Autodesk Inventor part; units mm, degrees
ref_plane "YZ Plane" through (0, 0, 0) normal (1, 0, 0) x (0, 1, 0)
ref_plane "XZ Plane" through (0, 0, 0) normal (0, 1, 0) x (-1, 0, 0)
ref_plane "XY Plane" through (0, 0, 0) normal (0, 0, 1) x (1, 0, 0)
sketch "Boceto1" plane through (0, 0, 0) normal (0, 1, 0) x (-1, 0, 0)
  arc A0 (16, 0) -> (-16, 0) centre (0, 0) ccw
  line L0 (0, 0) -> (45, 0) construction
  arc A1 (-16, -45) -> (16, -45) centre (0, -45) ccw
  line L1 (16, 0) -> (16, -45)
  line L2 (-16, -45) -> (-16, 0)
  arc A2 (15, 0) -> (-15, 0) centre (0, 0) ccw
  arc A3 (-15, -45) -> (15, -45) centre (0, -45) ccw
  line L3 (15, 0) -> (15, -45)
  line L4 (-15, -45) -> (-15, 0)
  dimension "d0" = 32
  dimension "d3" = 32
  dimension "d4" = 30
  dimension "d5" = 30
extrude "Extrusión1" add sketch "Boceto1" along normal blind 38
properties part number "Cinta"
CAD build for the part. Positions are in the model's coordinates, mm. A direction names the side the tool comes from. Give positions to 0.01 mm unless a question says otherwise; leave off trailing zeros. Loops run counter-clockwise (first coordinate to the right, second up) from the corner with the lowest first, then second, coordinate; pieces in that order, holes last. Notation, with made-up numbers: M 86,38.5 L 98,38.5 A6 ccw 98,42.5 Z; hole C 49,40.25 d11. An arc over 180 degrees is marked long. One line per question, with ' | ' between items. Start each with the question number.
1. Saw through at B-B on y = 3.5. Give the cut face in (x, z).
2. Two-plate mould, pull along Z, no slides. Class faces 3 (the face through (0, 19, 16)), 4 (the face through (0, 19, 15)), 5 (the face through (-15.3, 38, -19.5)): pulls with the +Z half, pulls with the -Z half, needs draft (parallel to the pull), parting line crosses it, or undercut.
3. Saw through at C-C on x = 7. Give the cut face in (y, z), plus the area to 3 significant figures.
4. Saw through at A-A on z = -38.5. Give the cut face in (x, y).
5. Probe L1, parallel to X at y = 17, z = -25; L2, parallel to Z at x = -5, y = 12; L3, parallel to X at y = 8.5, z = 2. List the from-to ranges inside material, lowest first. Write a range as from..to.
6. Flat gauge pins, fed straight in: pin 1 (12 mm diameter, centred on x = 13, y = 26, fed in from +Z); pin 2 (6 mm diameter, centred on x = -9.5, y = 4.5, fed in from +Z). Where does each tip first touch, or does it go through?
7. 3-axis set-ups, long thin cutter, end or side, ignore diameter. For faces 1 (the face through (16, 19, -23)), 2 (the face through (-15, 19, -22)): which of +Z, -Z, +X, -X, +Y, -Y reach the whole face in a straight line?
Result sheet:
1) outline: M -16,-45 A16 ccw 16,-45 L 16,0 A16 ccw -16,0 Z; hole M -15,-45 A15 ccw 15,-45 L 15,0 A15 ccw -15,0 Z
2) face 3: pulls with the +Z half | face 4: undercut | face 5: needs draft
3) outline: M 0,-59.39 L 38,-59.39 L 38,-58.27 L 0,-58.27 Z; M 0,13.27 L 38,13.27 L 38,14.39 L 0,14.39 Z | area: 85.2 mm^2
4) outline: M -16,0 L -15,0 L -15,38 L -16,38 Z; M 15,0 L 16,0 L 16,38 L 15,38 Z
5) L1: x = -16..-15, 15..16 | L2: z = -60.2..-59.14, 14.14..15.2 | L3: x = -15.87..-14.87, 14.87..15.87
6) pin 1: stops at z = 14.39 | pin 2: stops at z = 14.62
7) face 1: +Z, -Z, +X, +Y, -Y | face 2: +Y, -Y
